```python
from build123d import *

# Parameters (mm, degrees)
SKETCH1_W           = 15.8
SKETCH1_H           = 7.9
BOSS_EXTRUDE1_DEPTH = 3.2
SKETCH2_W           = 1.507644264
SKETCH2_H           = 1.6
CUT_EXTRUDE1_DEPTH  = 15.8


with BuildPart() as part:
    # Sketch1 → Boss-Extrude1 (new body)
    with BuildSketch(Plane(origin=(0, 0, 0), x_dir=(1, 0, 0), z_dir=(0, 1, 0))):
        with Locations((7.9, 3.95)):
            Rectangle(SKETCH1_W, SKETCH1_H)
    extrude(amount=BOSS_EXTRUDE1_DEPTH)

    # Sketch2 → Cut-Extrude1 (cut)
    with BuildSketch(Plane.ZY):
        with Locations((-2.382059289, 2.4)):
            Rectangle(SKETCH2_W, SKETCH2_H)
        with Locations((-5.517940711, 2.4)):
            Rectangle(SKETCH2_W, SKETCH2_H)
    extrude(amount=-CUT_EXTRUDE1_DEPTH, mode=Mode.SUBTRACT)


solid = part.part
```
The listing builds one solid part. Answer for the finished solid, in the listing's coordinates (mm). A direction names the side the tool comes from. Round coordinates to 2 decimals unless told otherwise and drop trailing zeros. Loops run counter-clockwise (first coordinate to the right, second up) from the corner with the lowest first, then second, coordinate; pieces in that order, holes last.
Q1. Section B-B, the plane x = 8 is taken. Determine the outline of the cut face in (y, z).
Q2. Section C-C, the plane z = -5.25 is taken. Determine the outline of the cut face in (x, y), then the cut area to 3 significant figures.
Q3. Find the intervals of material crossed by line 1 (Z direction, x = 5.5, y = 2.4); line 2 (Y direction, x = 4.75, z = -2.75), in increasing order.
Q4. Which of the six approach directions +Z, -Z, +X, -X, +Y, -Y give full straight-line access (tool end or side, diameter ignored) to faces 1 (the face through (8, 2, -4.764)), 2 (the face through (8, 2, 0))?
Q5. Section A-A, the plane y = 2.15 is taken. Determine the outline of the cut face in (x, z), then the cut area to 3 significant figures.
Q6. Given pin 1 Ø0.5 at (x, z) = (9.5, -2.5) entering from +Y, flat-ended and moving along its own axis, determine where the tip first touches the part or whether it passes through.
Completed:
1. outline: (0, -7.9) - (3.2, -7.9) - (3.2, -6.27) - (1.6, -6.27) - (1.6, -4.76) - (3.2, -4.76) - (3.2, -3.14) - (1.6, -3.14) - (1.6, -1.63) - (3.2, -1.63) - (3.2, 0) - (0, 0) - close
2. outline: (0, 0) - (15.8, 0) - (15.8, 1.6) - (0, 1.6) - close
2. area: 25.3 mm2
3. line 1: z = -7.9 to -6.27, -4.76 to -3.14, -1.63 to 0
3. line 2: y = 0 to 1.6
4. face 1: +X, -X, +Y
4. face 2: +Z, +X, -X, +Y, -Y
5. outline: (0, -7.9) - (15.8, -7.9) - (15.8, -6.27) - (0, -6.27) - close; (0, -4.76) - (15.8, -4.76) - (15.8, -3.14) - (0, -3.14) - close; (0, -1.63) - (15.8, -1.63) - (15.8, 0) - (0, 0) - close
5. area: 77.2 mm2
6. pin 1: stops at y = 1.6
